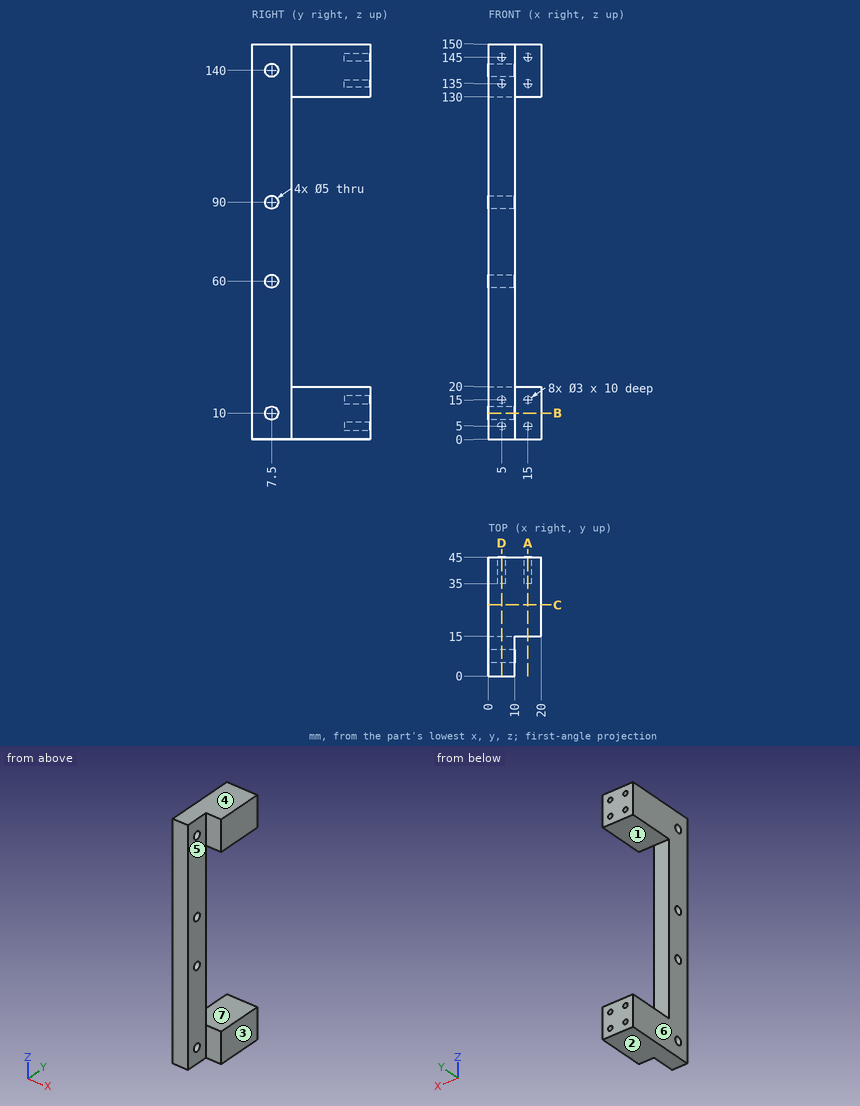
Verification items for this drawing (mm, ordinates from the low corner). A direction names the side the tool comes from. Give positions to 0.01 mm unless a question says otherwise; leave off trailing zeros. Write each loop counter-clockwise with the first axis right and the second up, starting at its lowest first coordinate (ties: lowest second). Pieces come first, ordered by that corner, then holes. Notation, with made-up numbers: (18.25, -13.5) - (67.25, -13.5) arc R16 cw to (67.25, 2.5) - close; hole circle Ø1 at (57, 69). An arc over 180 degrees is marked (long way). Answer as CSV lines item,"result". Start each with the question number.
1. Sectioned sample at D-D (x = 5). Record the boundary of the cut face in (y, z).
2. Sectioned sample at A-A (x = 15). Record the boundary of the cut face in (y, z).
3. Draft check along Z on the marked faces 1, 2, 3 and 4. Enter one of: pulls with the +Z half, pulls with the -Z half, needs draft (parallel to the pull), parting line crosses it, or undercut.
4. Set-up check for the marked faces 5, 6 and 7: record each of +Z, -Z, +X, -X, +Y, -Y from which the full face is reachable in a straight line by a thin tool's end or side.
5. Thickness scan on line 1 (X direction, y = 42, z = 135); line 2 (Z direction, x = 15.25, y = 39); line 3 (Z direction, x = 11.5, y = 21.5). Record the ranges inside material, lowest first.
6. Sectioned sample at C-C (y = 27). Record the boundary of the cut face in (x, z).
7. Sectioned sample at B-B (z = 10). Record the boundary of the cut face in (x, y), then the cut area to 3 significant figures.
8. Depth check by flat-ended pin: pin 1 (1.5 mm diameter, centred on x = 5, z = 135.5, fed in from +Y); pin 2 (11 mm diameter, centred on x = 4, z = 47.5, fed in from +Y); pin 3 (2.5 mm diameter, centred on x = 15, z = 5, fed in from -Y). Enter the tip coordinate at first touch or a pass-through.
Derived:
1,outline,"(0, 0) - (45, 0) - (45, 3.5) - (35, 3.5) - (35, 6.5) - (45, 6.5) - (45, 13.5) - (35, 13.5) - (35, 16.5) - (45, 16.5) - (45, 20) - (15, 20) - (15, 130) - (45, 130) - (45, 133.5) - (35, 133.5) - (35, 136.5) - (45, 136.5) - (45, 143.5) - (35, 143.5) - (35, 146.5) - (45, 146.5) - (45, 150) - (0, 150) - close; hole circle Ø5 at (7.5, 10); hole circle Ø5 at (7.5, 60); hole circle Ø5 at (7.5, 90); hole circle Ø5 at (7.5, 140)"
2,outline,"(15, 0) - (45, 0) - (45, 3.5) - (35, 3.5) - (35, 6.5) - (45, 6.5) - (45, 13.5) - (35, 13.5) - (35, 16.5) - (45, 16.5) - (45, 20) - (15, 20) - close; (15, 130) - (45, 130) - (45, 133.5) - (35, 133.5) - (35, 136.5) - (45, 136.5) - (45, 143.5) - (35, 143.5) - (35, 146.5) - (45, 146.5) - (45, 150) - (15, 150) - close"
3,face 1,"undercut"
3,face 2,"pulls with the -Z half"
3,face 3,"needs draft"
3,face 4,"pulls with the +Z half"
4,face 5,"+Z, -Z, +X, -Y"
4,face 6,"+Z, -Z, -X, +Y, -Y"
4,face 7,"+X, -X, +Y"
5,line 1,"0 to 3.5, 6.5 to 13.5, 16.5 to 20"
5,line 2,"0 to 3.52, 6.48 to 13.52, 16.48 to 20, 130 to 133.52, 136.48 to 143.52, 146.48 to 150"
5,line 3,"0 to 20, 130 to 150"
6,outline,"(0, 0) - (20, 0) - (20, 20) - (0, 20) - close; (0, 130) - (20, 130) - (20, 150) - (0, 150) - close"
7,outline,"(0, 0) - (10, 0) - (10, 5) - (0, 5) - close; (0, 10) - (10, 10) - (10, 15) - (20, 15) - (20, 45) - (0, 45) - close"
7,area,"700 mm²"
8,pin 1,"y = 35"
8,pin 2,"y = 15"
8,pin 3,"y = 15"
